Design review of the part shown in the three views and the two pictorial views. Dimensions are in mm from the part's minimum x, y and z. A direction names the side the tool comes from. Coordinates: 2 decimals unless noted, no trailing zeros. Loops run counter-clockwise (first coordinate to the right, second up) from the corner with the lowest first, then second, coordinate; pieces in that order, holes last. Notation, with made-up numbers: (-20, 80) -> (-6, 80) arc R19 ccw to (-6, 92) -> close; hole circle Ø9 at (69, 56). An arc over 180 degrees is marked (long way). Use a Markdown table: item, result. Add a question column.
Q1. For probe 1 along X at (y, z) = (9.25, 6.7); probe 2 along Z at (x, y) = (6.7, 3.5); probe 3 along X at (y, z) = (10, 8), list the stretches that pass through material, from the lowest coordinate up.
Q2. Draft analysis for pull direction X (two halves, no side actions). For the marked faces 1, 2 and 3, state which applies: pulls with the +X half, pulls with the -X half, needs draft (parallel to the pull), parting line crosses it, or undercut.
Q3. Take a section at C-C on x = 4.5. Write out the cut boundary in (y, z).
Q4. For the marked faces 4 and 5, list the 3-axis set-ups (+Z, -Z, +X, -X, +Y, -Y) from which the entire face can be reached by the end or side of a thin tool; tool diameter is ignored.
Q5. Take a section at B-B on z = 6.7. Write out the cut boundary in (x, y).
Q6. Take a section at D-D on y = 5.75. Write out the cut boundary in (x, z), plus the area to 3 significant figures.
Q7. Take a section at A-A on x = 6.7. Write out the cut boundary in (y, z).
Q8. Clearance check with flat-ended pins moving along their axes: pin 1 Ø1.5 at (x, y) = (9, 12.5) entering from +Z; pin 2 Ø1.9 at (x, z) = (6.7, 6.7) entering from -Y; pin 3 Ø4 at (y, z) = (3.77, 6.7) entering from +X; pin 4 Ø1.5 at (y, z) = (2, 6.5) entering from -X. State where each tip first meets the part, or that it passes through.
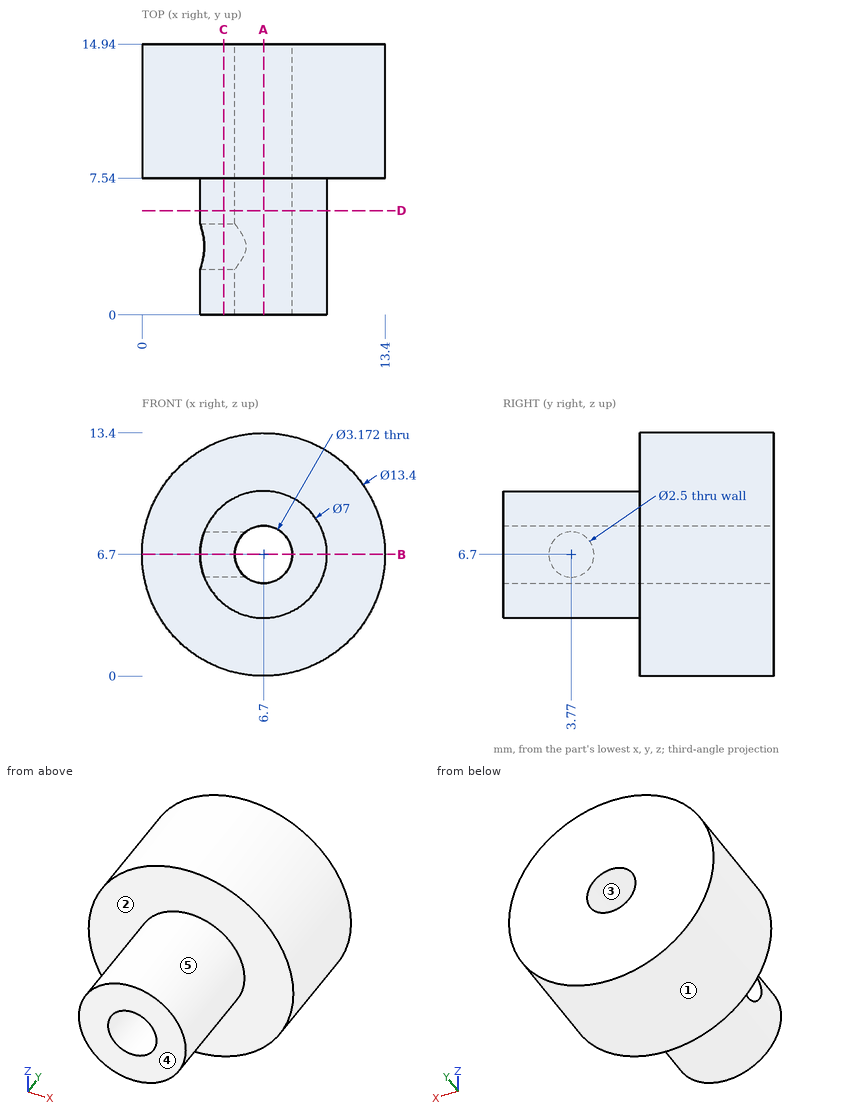
Answer list:
| question | item | result |
|---|---|---|
| 1 | probe 1 | 0 to 5.11, 8.29 to 13.4 |
| 1 | probe 2 | 3.2 to 5.11, 8.29 to 10.2 |
| 1 | probe 3 | 0.13 to 5.79, 7.61 to 13.27 |
| 2 | face 1 | parting line crosses it |
| 2 | face 2 | needs draft |
| 2 | face 3 | undercut |
| 3 | outline | (0, 3.98) -> (7.54, 3.98) -> (7.54, 0.37) -> (14.94, 0.37) -> (14.94, 13.03) -> (7.54, 13.03) -> (7.54, 9.42) -> (0, 9.42) -> close; hole circle Ø2.5 at (3.77, 6.7) |
| 4 | face 4 | +Z, -Z, +X, -X, -Y |
| 4 | face 5 | -Y |
| 5 | outline | (0, 7.54) -> (3.2, 7.54) -> (3.2, 5.02) -> (5.11, 5.02) -> (5.11, 14.94) -> (0, 14.94) -> close; (3.2, 0) -> (5.11, 0) -> (5.11, 2.52) -> (3.2, 2.52) -> close; (8.29, 0) -> (10.2, 0) -> (10.2, 7.54) -> (13.4, 7.54) -> (13.4, 14.94) -> (8.29, 14.94) -> close |
| 6 | outline | circle Ø7 at (6.7, 6.7); hole circle Ø3.17 at (6.7, 6.7) |
| 6 | area | 30.6 mm² |
| 7 | outline | (0, 3.2) -> (7.54, 3.2) -> (7.54, 0) -> (14.94, 0) -> (14.94, 5.11) -> (0, 5.11) -> close; (0, 8.29) -> (14.94, 8.29) -> (14.94, 13.4) -> (7.54, 13.4) -> (7.54, 10.2) -> (0, 10.2) -> close |
| 8 | pin 1 | z = 13.22 |
| 8 | pin 2 | through |
| 8 | pin 3 | x = 10.2 |
| 8 | pin 4 | x = 3.2 |
